The listing builds one solid part. Answer for the finished solid, in the listing's coordinates (mm). Round coordinates to 2 decimals unless told otherwise and drop trailing zeros. Order: outer loops, then holes, each group sorted by start corner. A loop starts at its lowest first (then second) coordinate and runs counter-clockwise, first axis right, second up. Notation, with made-up numbers: (-18.75, 42.25) -> (34.25, 42.25) arc R19 ccw to (34.25, 50.25) -> close; hole circle Ø8 at (37.5, 65). An arc over 180 degrees is marked (long way). Answer in a Markdown table with one row per item. Add a question column.
```python
from build123d import *

# Parameters (mm, degrees)
SKETCH1_R           = 88.365
SKETCH1_R_2         = 85.865
BOSS_EXTRUDE1_DEPTH = 42.425
SKETCH2_W           = 20
SKETCH2_H           = 11
CUT_EXTRUDE1_DEPTH  = 89.365
CIRPATTERN1_COUNT   = 13


with BuildPart() as part:
    # Sketch1 → Boss-Extrude1 (new body)
    with BuildSketch(Plane(origin=(0, 0, 0), x_dir=(1, 0, 0), z_dir=(0, 1, 0))):
        Circle(SKETCH1_R)
        Circle(SKETCH1_R_2, mode=Mode.SUBTRACT)
    extrude(amount=BOSS_EXTRUDE1_DEPTH)

    # Sketch2 → Cut-Extrude1 (cut, symmetric)
    with BuildSketch(Plane.XY):
        with Locations((0, 19.5)):
            Rectangle(SKETCH2_W, SKETCH2_H)
    cut_extrude1 = extrude(amount=CUT_EXTRUDE1_DEPTH, both=True, mode=Mode.SUBTRACT)

    # CirPattern1: Cut-Extrude1 ×13 about axis
    cirpattern1_axis = Axis((0, 0, 0), (0, 1, 0))
    for i in range(1, CIRPATTERN1_COUNT):
        add(cut_extrude1.rotate(cirpattern1_axis, i * 360 / CIRPATTERN1_COUNT), mode=Mode.SUBTRACT)


solid = part.part
```
1. The part is cut by section C-C (y = 33.5). Give the vertices of the cut face in (x, z) (3 decimals).
2. The mould has two halves that part along Z. Classify faces 1 (the flat face through (81, 25, 31)), 2 (the flat face through (86, 14, 11)): released by +Z, released by -Z, zero draft, split by the parting line, or undercut.
3. Each of these flat-tipped pins is pushed along its axis until it touches: pin 1 (2 mm diameter, centred on x = 34, y = 6.5, fed in from -Z); pin 2 (1 mm diameter, centred on y = 13, z = 13.5, fed in from -X); pin 3 (0.8 mm diameter, centred on y = 18.5, z = 86.5, fed in from +X). Where does it stop, or does it pass through?
4. Straight lines are drawn through the part: line 1 along X through (y, z) = (24, 0) (3 decimals); line 2 along X through (y, z) = (9.5, 40). For each, find the intervals that lie inside material, in ascending order.
5. The part is cut by section A-A (x = 0). Give the vertices of the cut face in (y, z) (3 decimals), then the cut area to 3 significant figures.
6. The part is cut by section B-B (z = 68). Give the vertices of the cut face in (x, y) (3 decimals).
Report:
| question | item | result |
|---|---|---|
| 1 | outline | circle Ø176.73 at (0, 0); hole circle Ø171.73 at (0, 0) |
| 2 | face 1 | undercut |
| 2 | face 2 | undercut |
| 3 | pin 1 | stops at z = -81.97 |
| 3 | pin 2 | stops at x = -87.4 |
| 3 | pin 3 | stops at x = 11.12 |
| 4 | line 1 | x = -88.365 to -85.865, 85.865 to 88.365 |
| 4 | line 2 | x = -78.79 to -75.98, 75.98 to 78.79 |
| 5 | outline | (0, -88.365) -> (14, -88.365) -> (14, -85.865) -> (0, -85.865) -> close; (0, 85.865) -> (14, 85.865) -> (14, 88.365) -> (0, 88.365) -> close; (25, -88.365) -> (42.425, -88.365) -> (42.425, -85.865) -> (25, -85.865) -> close; (25, 85.865) -> (42.425, 85.865) -> (42.425, 88.365) -> (25, 88.365) -> close |
| 5 | area | 157 mm^2 |
| 6 | outline | (-56.43, 0) -> (-52.429, 0) -> (-52.429, 14) -> (-56.43, 14) -> close; (-56.43, 25) -> (-52.429, 25) -> (-52.429, 42.425) -> (-56.43, 42.425) -> close; (52.429, 0) -> (56.43, 0) -> (56.43, 14) -> (52.429, 14) -> close; (52.429, 25) -> (56.43, 25) -> (56.43, 42.425) -> (52.429, 42.425) -> close |
